CAD build for the part. Positions are in the model's coordinates, mm. Coordinates: 2 decimals unless noted, no trailing zeros. Loops run counter-clockwise (first coordinate to the right, second up) from the corner with the lowest first, then second, coordinate; pieces in that order, holes last. Notation, with made-up numbers: (52.25, 25.5) -> (62.25, 25.5) arc R15 cw to (62.25, 54.5) -> close; hole circle Ø8 at (9, -4.75). An arc over 180 degrees is marked (long way). Answer as a JSON object with one key per item and string values. Group by question number.
from build123d import *

# Parameters (mm, degrees)
SKETCH1_R           = 65
SKETCH1_R_2         = 1.65
SKETCH1_R_3         = 2.5
SKETCH1_R_4         = 1.5
BOSS_EXTRUDE1_DEPTH = 5


with BuildPart() as part:
    # Sketch1 → Boss-Extrude1 (new body)
    with BuildSketch(Plane.XY):
        Circle(SKETCH1_R)
        with Locations((0, 55)):
            Circle(SKETCH1_R_2, mode=Mode.SUBTRACT)
        with Locations((47.631397208, 27.5)):
            Circle(SKETCH1_R_2, mode=Mode.SUBTRACT)
        with Locations((47.631397208, -27.5)):
            Circle(SKETCH1_R_2, mode=Mode.SUBTRACT)
        with Locations((0, -55)):
            Circle(SKETCH1_R_2, mode=Mode.SUBTRACT)
        with Locations((-47.631397208, -27.5)):
            Circle(SKETCH1_R_2, mode=Mode.SUBTRACT)
        with Locations((-47.631397208, 27.5)):
            Circle(SKETCH1_R_2, mode=Mode.SUBTRACT)
        with Locations((0, 27)):
            Circle(SKETCH1_R_3, mode=Mode.SUBTRACT)
        with Locations((6.062177826, 23.5)):
            Circle(SKETCH1_R_3, mode=Mode.SUBTRACT)
        with Locations((6.062177826, 16.5)):
            Circle(SKETCH1_R_3, mode=Mode.SUBTRACT)
        with Locations((0, 13)):
            Circle(SKETCH1_R_3, mode=Mode.SUBTRACT)
        with Locations((-6.062177826, 16.5)):
            Circle(SKETCH1_R_3, mode=Mode.SUBTRACT)
        with Locations((-6.062177826, 23.5)):
            Circle(SKETCH1_R_3, mode=Mode.SUBTRACT)
        with Locations((0, 20)):
            Circle(SKETCH1_R_4, mode=Mode.SUBTRACT)
        with Locations(Location((6.062177826, -16.5, 0), (0, 0, 180))):
            Circle(SKETCH1_R_3, mode=Mode.SUBTRACT)
        with Locations(Location((0, -13, 0), (0, 0, 180))):
            Circle(SKETCH1_R_3, mode=Mode.SUBTRACT)
        with Locations(Location((-6.062177826, -16.5, 0), (0, 0, 180))):
            Circle(SKETCH1_R_3, mode=Mode.SUBTRACT)
        with Locations(Location((0, -20, 0), (0, 0, 180))):
            Circle(SKETCH1_R_4, mode=Mode.SUBTRACT)
        with Locations(Location((-6.062177826, -23.5, 0), (0, 0, 180))):
            Circle(SKETCH1_R_3, mode=Mode.SUBTRACT)
        with Locations(Location((0, -27, 0), (0, 0, 180))):
            Circle(SKETCH1_R_3, mode=Mode.SUBTRACT)
        with Locations(Location((6.062177826, -23.5, 0), (0, 0, 180))):
            Circle(SKETCH1_R_3, mode=Mode.SUBTRACT)
    extrude(amount=BOSS_EXTRUDE1_DEPTH)


solid = part.part
Item 1: Band-saw the part on A-A, the plane z = 1.6. Count the separate pieces of the cut face and the enclosed holes in it, and give its area (3 significant figures).
Item 2: Band-saw the part on B-B, the plane y = 55. List the corners of the cut face in (x, z).
Item 3: Drill centre lines: L1, parallel to Y at x = 8, z = 0.3; L2, parallel to X at y = -16.5, z = 3.4; L3, parallel to X at y = 16, z = 2. Where is each one in solid material? Low to high.
Item 4: Band-saw the part on D-D, the plane x = -24. List the corners of the cut face in (y, z).
Item 5: Pull direction Y, two halves, no side cores. Call faces 1 (the cylindrical face through (62, 19.52, 2.46)), 2 (the flat face through (-1, 1, 0)), 3 (the cylindrical face through (48.52, 28.89, 2.46)): +Y half, -Y half, draft (parallel to the pull), parting line (faces both ways), or undercut.
Item 6: Flat gauge pins, fed straight in: P1, Ø4, axis at x = 0, y = 55, coming from the -Z side; P2, Ø1.8, axis at x = 0, y = 20, coming from the +Z side; P3, Ø1, axis at x = -39.5, z = 3.5, coming from the -Y side. Where does each tip first touch, or does it go through?
Reply:
{
 "1": {"separate pieces": "1", "enclosed holes": "20", "area": "13,000 mm²"},
 "2": {"outline": "(-34.64, 0) -> (-1.65, 0) -> (-1.65, 5) -> (-34.64, 5) -> close; (1.65, 0) -> (34.64, 0) -> (34.64, 5) -> (1.65, 5) -> close"},
 "3": {"L1": "-64.51 to -25.08, -21.92 to -18.08, -14.92 to 14.92, 18.08 to 21.92, 25.08 to 64.51", "L2": "-62.87 to -8.56, -3.56 to 3.56, 8.56 to 62.87", "L3": "-63 to -8.51, -3.61 to 3.61, 8.51 to 63"},
 "4": {"outline": "(-60.41, 0) -> (60.41, 0) -> (60.41, 5) -> (-60.41, 5) -> close"},
 "5": {"face 1": "parting line", "face 2": "draft", "face 3": "undercut"},
 "6": {"P1": "z = 0", "P2": "through", "P3": "y = -52"}
}
